The listing builds one solid part. Answer for the finished solid, in the listing's coordinates (mm). A direction names the side the tool comes from. Coordinates: 2 decimals unless noted, no trailing zeros. Order: outer loops, then holes, each group sorted by start corner. A loop starts at its lowest first (then second) coordinate and runs counter-clockwise, first axis right, second up.
from build123d import *

# Parameters (mm, degrees)
BOSS_EXTRUDE1_DEPTH = 20
SKETCH2_W           = 35
SKETCH2_H           = 25
CUT_EXTRUDE1_DEPTH  = 10
CUT_EXTRUDE2_START  = 20
SKETCH3_R           = 11.1
CUT_EXTRUDE2_DEPTH  = 25
SKETCH4_R           = 5
CUT_EXTRUDE3_DEPTH  = 6
SKETCH5_R           = 2.75
CUT_EXTRUDE4_DEPTH  = 26


with BuildPart() as part:
    # Sketch1 → Boss-Extrude1 (new body)
    with BuildSketch(Plane(origin=(0, 0, 0), x_dir=(1, 0, 0), z_dir=(0, 1, 0))):
        Polygon((0, 0), (60, 0), (60, 35), (20, 35), (20, 15), (0, 15), align=None)
    extrude(amount=BOSS_EXTRUDE1_DEPTH)

    # Sketch2 → Cut-Extrude1 (cut)
    with BuildSketch(Plane(origin=(0, 20, 0), x_dir=(1, 0, 0), z_dir=(0, 1, 0))):
        with Locations((42.5, 22.5)):
            Rectangle(SKETCH2_W, SKETCH2_H)
    extrude(amount=-CUT_EXTRUDE1_DEPTH, mode=Mode.SUBTRACT)

    # Sketch3 → Cut-Extrude2 (cut)
    with BuildSketch(Plane(origin=(0, 10, 0), x_dir=(1, 0, 0), z_dir=(0, 1, 0)).offset(CUT_EXTRUDE2_START)):
        with Locations((46.1, 12.525762493)):
            Circle(SKETCH3_R)
    extrude(amount=-CUT_EXTRUDE2_DEPTH, mode=Mode.SUBTRACT)

    # Sketch4 → Cut-Extrude3 (cut, through all)
    with BuildSketch(Plane(origin=(0, 5, 0), x_dir=(1, 0, 0), z_dir=(0, 1, 0))):
        with Locations((46.1, 12.525762493)):
            Circle(SKETCH4_R)
    extrude(amount=-CUT_EXTRUDE3_DEPTH, mode=Mode.SUBTRACT)

    # Sketch5 → Cut-Extrude4 (cut, through all)
    with BuildSketch(Plane(origin=(25, 0, 0), x_dir=(0, 0, -1), z_dir=(1, 0, 0))):
        with Locations((25, 14)):
            Circle(SKETCH5_R)
    extrude(amount=-CUT_EXTRUDE4_DEPTH, mode=Mode.SUBTRACT)


solid = part.part
1) A tool of negligible diameter and unlimited length cuts with its end or side. For faces 1 (the face through (43.69, 10.94, -1.69)), 2 (the face through (0, 10, -8)), 3 (the face through (20, 10, -25)), 4 (the face through (42, 10, -25)), from which of +Z, -Z, +X, -X, +Y, -Y can it reach the whole face along a straight path? Write none if from no direction.
2) Consider L1, parallel to Z at x = 46.1, y = 8.75; L2, parallel to Y at x = 46, z = -30; L3, parallel to Z at x = 17, y = 11.75. Determine where each line is inside the solid, lowest interval first.
3) Each of these flat-tipped pins is pushed along its axis until it touches: P1, Ø2, axis at x = 18, y = 5, coming from the -Z side; P2, Ø11, axis at y = 15, z = -17, coming from the +X side; P3, Ø9, axis at x = 46.1, z = -12.53, coming from the +Y side; P4, Ø3, axis at x = 28, y = 17, coming from the -Z side. Where does it stop, or does it pass through?
4) Section C-C (y = 14) is taken. Give the vertices of the cut face in (x, z), then the cut area to 3 significant figures.
5) Section B-B (x = 46.1) is taken. Give the vertices of the cut face in (y, z), then the cut area to 3 significant figures.
6) Section A-A (z = -25) is taken. Give the vertices of the cut face in (x, y).
7) Determine the mould class of faces 5 (the face through (22.535, 14.121, -22.253)), 6 (the face through (21, 20, -9)), 7 (the face through (36, 0, -18)), 8 (the face through (58, 15, -10)) for opening direction Y: released by +Y, released by -Y, zero draft, split by the parting line, or undercut.
8) Section D-D (x = 21) is taken. Give the vertices of the cut face in (y, z).
Filled sheet:
1. face 1: +Y
1. face 2: +Z, -Z, -X, +Y, -Y
1. face 3: -Z, -X, +Y, -Y
1. face 4: -Z, +X, +Y
2. L1: z = -35 to -23.63, -1.43 to 0
2. L2: y = 0 to 10
2. L3: z = -15 to 0
3. P1: stops at z = -15
3. P2: stops at x = 60
3. P3: passes through
3. P4: stops at z = -10
4. outline: (0, -15) - (20, -15) - (20, -22.25) - (25, -22.25) - (25, -10) - (35.29, -10) arc R11.1 cw to (56.91, -10) - (60, -10) - (60, 0) - (0, 0) - close; (20, -35) - (25, -35) - (25, -27.75) - (20, -27.75) - close
4. area: 660 mm2
5. outline: (0, -35) - (10, -35) - (10, -23.63) - (5, -23.63) - (5, -17.53) - (0, -17.53) - close; (0, -7.53) - (5, -7.53) - (5, -1.43) - (20, -1.43) - (20, 0) - (0, 0) - close
5. area: 203 mm2
6. outline: (20, 0) - (60, 0) - (60, 10) - (25, 10) - (25, 11.25) - (20, 11.25) - close; (20, 16.75) - (25, 16.75) - (25, 20) - (20, 20) - close
7. face 5: undercut
7. face 6: released by +Y
7. face 7: released by -Y
7. face 8: zero draft
8. outline: (0, -35) - (20, -35) - (20, 0) - (0, 0) - close; hole circle Ø5.5 at (14, -25)
